Could you check a few things on this model? Use its own coordinates, in mm. Round coordinates to 2 decimals unless told otherwise and drop trailing zeros. Loops run counter-clockwise (first coordinate to the right, second up) from the corner with the lowest first, then second, coordinate; pieces in that order, holes last.
from build123d import *

# Parameters (mm, degrees)
BOSS_EXTRUDE1_DEPTH     = 10
FILLET1_R               = 3
SKETCH2_R               = 1
CUT_EXTRUDE1_DEPTH      = 1
CUT_EXTRUDE1_DEPTH_BACK = 1.35


with BuildPart() as part:
    # Sketch1 → Boss-Extrude1 (new body)
    with BuildSketch(Plane(origin=(0, 0, 0), x_dir=(0, 0, -1), z_dir=(1, 0, 0))):
        with BuildLine():
            Line((0, 30), (0, 0))
            ThreePointArc((0, 0), (-0.025, -0.025), (-0.05, 0))
            Line((-0.05, 0), (-0.05, 30))
            Line((-0.05, 30), (-0.2, 30))
            Line((-0.2, 30), (-0.2, 0))
            ThreePointArc((-0.2, 0), (-0.025, -0.175), (0.15, 0))
            Line((0.15, 0), (0.15, 30))
            Line((0.15, 30), (0, 30))
        make_face()
    extrude(amount=BOSS_EXTRUDE1_DEPTH)

    # Fillet1
    fillet1_edges = [part.edges().sort_by_distance(p)[0] for p in [
        (0, 30, -0.075),
        (10, 30, 0.125),
        (10, 30, -0.075),
        (0, 30, 0.125),
    ]]
    fillet(fillet1_edges, radius=FILLET1_R)

    # Sketch2 → Cut-Extrude1 (cut, two sides)
    with BuildSketch(Plane.XY.offset(0.2)) as cut_extrude1_sk:
        with Locations((5, 24.25)):
            Circle(SKETCH2_R)
        with Locations((5, 5.75)):
            Circle(SKETCH2_R)
    extrude(amount=CUT_EXTRUDE1_DEPTH, mode=Mode.SUBTRACT)
    extrude(cut_extrude1_sk.sketch, amount=-CUT_EXTRUDE1_DEPTH_BACK, mode=Mode.SUBTRACT)


solid = part.part
Item 1: If I drill on line 1 along Y through (x, z) = (5, 0.1); line 2 along X through (y, z) = (23.5, -0.1); line 3 along Y through (x, z) = (7.75, 0.1), over which ranges is the centre line in solid material (lowest first)?
Results list:
line 1: y = -0.16 to 4.75, 6.75 to 23.25, 25.25 to 30
line 2: x = 0 to 4.34, 5.66 to 10
line 3: y = -0.16 to 29.9
Item 2: Will this pin go through, and if not, where does the flat tip stop? pin 1 (1.6 mm diameter, centred on x = 5, y = 5.75, fed in from +Z).
Results list:
pin 1: passes through
Item 3: If we section it at C-C, the plane x = 5: Please give me the cut outline in (y, z) (3 decimals).
Results list:
outline: (0, -0.15) - (4.75, -0.15) - (4.75, 0) - (0, 0) arc R0.025 cw to (0, 0.05) - (4.75, 0.05) - (4.75, 0.2) - (0, 0.2) arc R0.175 ccw to start; (6.75, -0.15) - (23.25, -0.15) - (23.25, 0) - (6.75, 0) - close; (6.75, 0.05) - (23.25, 0.05) - (23.25, 0.2) - (6.75, 0.2) - close; (25.25, -0.15) - (30, -0.15) - (30, 0) - (25.25, 0) - close; (25.25, 0.05) - (30, 0.05) - (30, 0.2) - (25.25, 0.2) - close
Item 4: If we section it at B-B, the plane y = 11: Please give me the cut outline in (x, z), then the cut area to 3 significant figures.
Results list:
outline: (0, -0.15) - (10, -0.15) - (10, 0) - (0, 0) - close; (0, 0.05) - (10, 0.05) - (10, 0.2) - (0, 0.2) - close
area: 3.00 mm2
Item 5: If we section it at D-D, the plane x = 2.25: Please give me the cut outline in (y, z) (3 decimals).
Results list:
outline: (0, -0.15) - (29.905, -0.15) - (29.905, 0) - (0, 0) arc R0.025 cw to (0, 0.05) - (29.905, 0.05) - (29.905, 0.2) - (0, 0.2) arc R0.175 ccw to start
Item 6: If we section it at A-A, the plane y = 24.25: Please give me the cut outline in (x, z).
Results list:
outline: (0, -0.15) - (4, -0.15) - (4, 0) - (0, 0) - close; (0, 0.05) - (4, 0.05) - (4, 0.2) - (0, 0.2) - close; (6, -0.15) - (10, -0.15) - (10, 0) - (6, 0) - close; (6, 0.05) - (10, 0.05) - (10, 0.2) - (6, 0.2) - close
